Verification items for this drawing (mm, ordinates from the low corner). A direction names the side the tool comes from. Give positions to 0.01 mm unless a question says otherwise; leave off trailing zeros. Write each loop counter-clockwise with the first axis right and the second up, starting at its lowest first coordinate (ties: lowest second). Pieces come first, ordered by that corner, then holes. Notation, with made-up numbers: (-20.5, 78) -> (24.5, 78) arc R21 cw to (24.5, 83) -> close; hole circle Ø11 at (84, -36). An arc over 180 degrees is marked (long way). One line per item, written item: value.
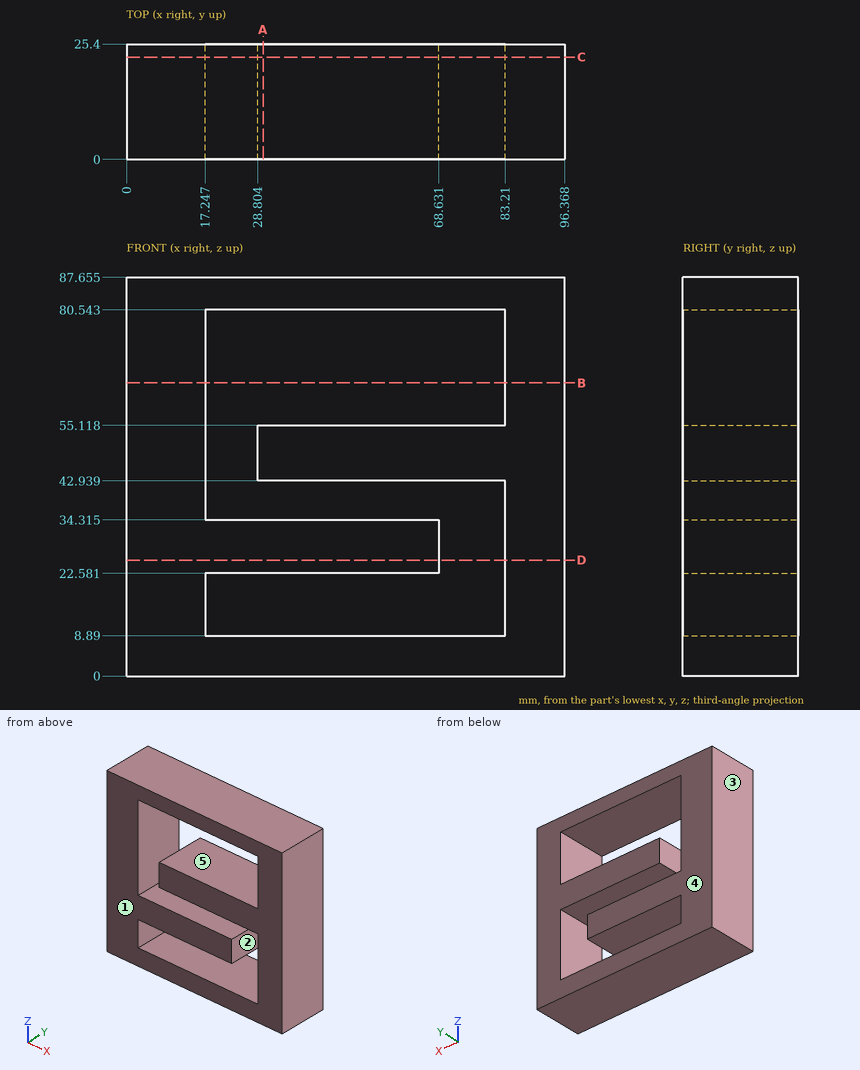
1) Sectioned sample at D-D on z = 25.5. Record the cut outline in (x, y).
Verdict:
outline: (0, 0) -> (68.63, 0) -> (68.63, 25.4) -> (0, 25.4) -> close; (83.21, 0) -> (96.37, 0) -> (96.37, 25.4) -> (83.21, 25.4) -> close
2) Sectioned sample at C-C on y = 22.5. Record the cut outline in (x, z) (1 decimal), plus the area to 3 significant figures.
Verdict:
outline: (0, 0) -> (96.4, 0) -> (96.4, 87.7) -> (0, 87.7) -> close; hole (17.2, 8.9) -> (83.2, 8.9) -> (83.2, 42.9) -> (28.8, 42.9) -> (28.8, 55.1) -> (83.2, 55.1) -> (83.2, 80.5) -> (17.2, 80.5) -> (17.2, 34.3) -> (68.6, 34.3) -> (68.6, 22.6) -> (17.2, 22.6) -> close
area: 4,990 mm^2
3) Mould release check, pull along X, two halves, no side actions. Record for the marked faces 3, 4 and 5: released by +X, released by -X, zero draft, split by the parting line, or undercut.
Verdict:
face 3: released by -X
face 4: zero draft
face 5: undercut
4) Scan lines: probe 1 along Z at (x, y) = (73.5, 12.5) (1 decimal); probe 2 along Z at (x, y) = (36.5, 6.75) (1 decimal); probe 3 along Z at (x, y) = (27, 7) (1 decimal). Record each from-to range of solid material in increasing order.
Verdict:
probe 1: 0 to 8.9, 42.9 to 55.1, 80.5 to 87.7
probe 2: 0 to 8.9, 22.6 to 34.3, 42.9 to 55.1, 80.5 to 87.7
probe 3: 0 to 8.9, 22.6 to 34.3, 80.5 to 87.7
5) Tool access check on the marked faces 1 and 2. Record the directions out of +Z, -Z, +X, -X, +Y, -Y that give a thin tool (end or side, any length) a straight path to the whole face; none if there is none.
Verdict:
face 1: +Z, -Z, +X, -X, -Y
face 2: +Y, -Y
6) Sectioned sample at B-B on z = 64.5. Record the cut outline in (x, y).
Verdict:
outline: (0, 0) -> (17.25, 0) -> (17.25, 25.4) -> (0, 25.4) -> close; (83.21, 0) -> (96.37, 0) -> (96.37, 25.4) -> (83.21, 25.4) -> close
7) Sectioned sample at A-A on x = 30. Record the cut outline in (y, z) (1 decimal), plus the area to 3 significant figures.
Verdict:
outline: (0, 0) -> (25.4, 0) -> (25.4, 8.9) -> (0, 8.9) -> close; (0, 22.6) -> (25.4, 22.6) -> (25.4, 34.3) -> (0, 34.3) -> close; (0, 42.9) -> (25.4, 42.9) -> (25.4, 55.1) -> (0, 55.1) -> close; (0, 80.5) -> (25.4, 80.5) -> (25.4, 87.7) -> (0, 87.7) -> close
area: 1,010 mm^2
